Autodesk Inventor part; units mm, degrees
ref_plane "YZ Plane" through (0, 0, 0) normal (1, 0, 0) x (0, 1, 0)
ref_plane "XZ Plane" through (0, 0, 0) normal (0, 1, 0) x (-1, 0, 0)
ref_plane "XY Plane" through (0, 0, 0) normal (0, 0, 1) x (1, 0, 0)
sketch "スケッチ1" plane through (0, 0, 0) normal (0, 0, 1) x (1, 0, 0)
  line L0 (0, 0) -> (45, 0)
  line L1 (45, 0) -> (45, 100)
  line L2 (45, 100) -> (0, 100)
  line L3 (0, 100) -> (0, 0)
  dimension "d0" = 100
  dimension "d1" = 45
extrude "押し出し1" add sketch "スケッチ1" along normal blind 10
sketch "スケッチ2" plane through (0, 0, 10) normal (0, 0, 1) x (1, 0, 0)
  line L0 (0, 0) -> (45, 0)
  point P0 (22.6447, 79.5)
  dimension "d4" = 79.5
hole "穴1" at (22.6447, 79.5, 10) direction (0, 0, -1) diameter 24 end through all
sketch "スケッチ3" plane through (0, 0, 0) normal (0, 0, -1) x (-1, 0, 0)
  line L0 (0, 0) -> (-45, 0)
  line L1 (-45, 0) -> (-45, 100)
  line L2 (0, 100) -> (0, 0)
  point P0 (-10, 10)
  point P1 (-35, 10)
  dimension "d12" = 10
  dimension "d13" = 10
  dimension "d14" = 10
  dimension "d15" = 10
hole "穴2" at (10, 10, 0) at (35, 10, 0) direction (0, 0, 1) diameter 5 end through all
properties part number "回転軸取り付け板"
CAD build for the part. Positions are in the model's coordinates, mm. Round coordinates to 2 decimals unless told otherwise and drop trailing zeros. Write each loop counter-clockwise with the first axis right and the second up, starting at its lowest first coordinate (ties: lowest second). Pieces come first, ordered by that corner, then holes.
Item 1: Band-saw the part on C-C on y = 86.5. Write the cut outline in (x, z), then the cut area to 3 significant figures.
Filled in:
outline: (0, 0) - (12.9, 0) - (12.9, 10) - (0, 10) - close; (32.39, 0) - (45, 0) - (45, 10) - (32.39, 10) - close
area: 255 mm2
Item 2: Band-saw the part on B-B on x = 31.5. Write the cut outline in (y, z), then the cut area to 3 significant figures.
Filled in:
outline: (0, 0) - (71.4, 0) - (71.4, 10) - (0, 10) - close; (87.6, 0) - (100, 0) - (100, 10) - (87.6, 10) - close
area: 838 mm2
Item 3: Drill centre lines: L1, parallel to X at y = 10, z = 3.5; L2, parallel to Y at x = 10, z = 6.75; L3, parallel to Y at x = 12, z = 9.25. Where is each one in solid material? Low to high.
Filled in:
L1: x = 0 to 7.5, 12.5 to 32.5, 37.5 to 45
L2: y = 0 to 7.5, 12.5 to 100
L3: y = 0 to 8.5, 11.5 to 73.96, 85.04 to 100
Item 4: Band-saw the part on A-A on y = 10. Write the cut outline in (x, z).
Filled in:
outline: (0, 0) - (7.5, 0) - (7.5, 10) - (0, 10) - close; (12.5, 0) - (32.5, 0) - (32.5, 10) - (12.5, 10) - close; (37.5, 0) - (45, 0) - (45, 10) - (37.5, 10) - close
Item 5: Band-saw the part on D-D on z = 7.75. Write the cut outline in (x, y).
Filled in:
outline: (0, 0) - (45, 0) - (45, 100) - (0, 100) - close; hole circle Ø5 at (10, 10); hole circle Ø24 at (22.64, 79.5); hole circle Ø5 at (35, 10)
Item 6: Drop a flat-ended pin along its axis: pin 1 Ø19 at (x, y) = (22.64, 79.5) entering from +Z. Give the stop position or say it passes through.
Filled in:
pin 1: passes through
Item 7: Mould opens along X. For faces 1 (the cylindrical face through (12.44, 9.46, 5.07)), 2 (the flat face through (45, 49, 5)), 3 (the flat face through (23, 100, 5)) say: released by +X, released by -X, zero draft, split by the parting line, or undercut.
Filled in:
face 1: undercut
face 2: released by +X
face 3: zero draft
